Check sheet for the drawn part. Datum: minimum x, y, z corner. Units: mm. Coordinates: 2 decimals unless noted, no trailing zeros. Order: outer loops, then holes, each group sorted by start corner. A loop starts at its lowest first (then second) coordinate and runs counter-clockwise, first axis right, second up. Notation, with made-up numbers: (13.5, -12) -> (67.5, -12) arc R23 ccw to (67.5, 8) -> close; hole circle Ø6 at (52, 24). An arc over 180 degrees is marked (long way). Answer as CSV lines item,"result".
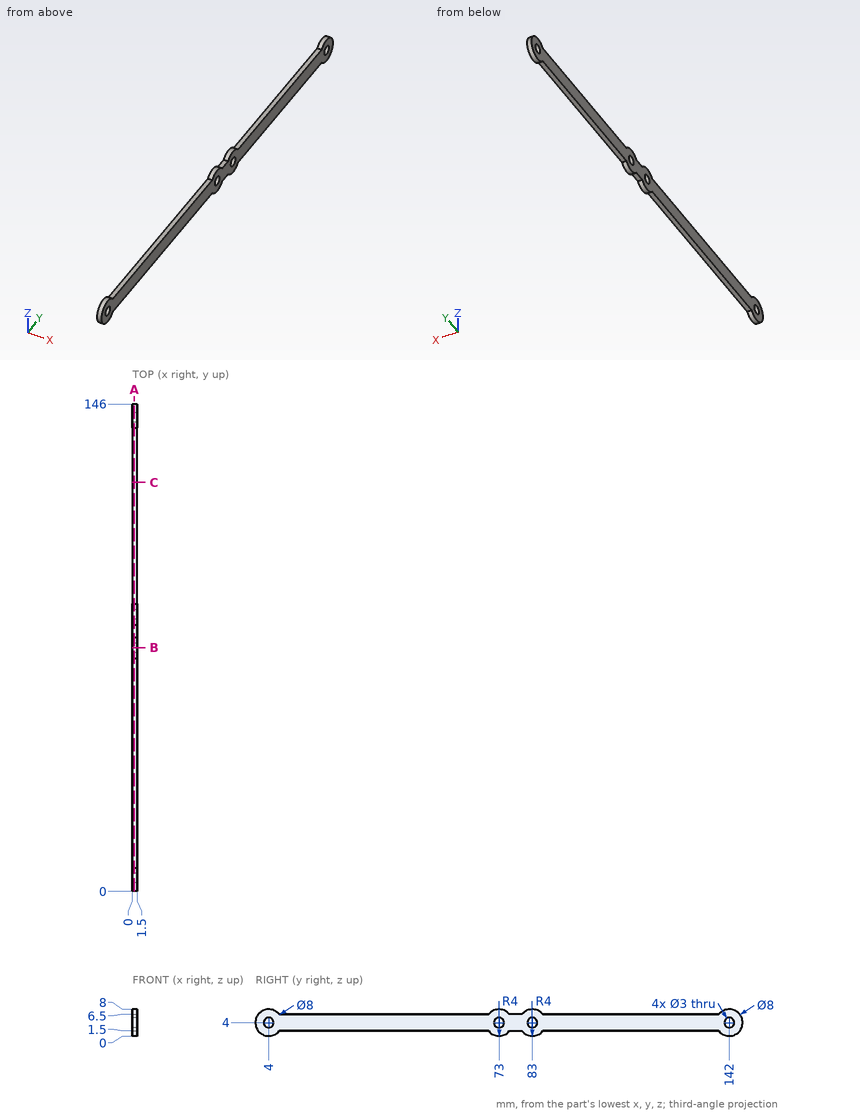
Item 1: Section check C-C, the plane y = 122.5. Record the boundary of the cut face in (x, z), plus the area to 3 significant figures.
Answer list:
outline,"(0, 1.5) -> (1.5, 1.5) -> (1.5, 6.5) -> (0, 6.5) -> close"
area,"7.50 mm2"
Item 2: Depth check by flat-ended pin: pin 1 Ø2.5 at (y, z) = (83, 4) entering from +X (3 decimals). Enter the tip coordinate at first touch or a pass-through.
Answer list:
pin 1,"through"
Item 3: Section check A-A, the plane x = 0.6. Record the boundary of the cut face in (y, z), plus the area to 3 significant figures.
Answer list:
outline,"(7.12, 1.5) -> (69.88, 1.5) arc R4 ccw to (76.12, 1.5) -> (79.88, 1.5) arc R4 ccw to (86.12, 1.5) -> (138.88, 1.5) arc R4 ccw (long way) to (138.88, 6.5) -> (86.12, 6.5) arc R4 ccw to (79.88, 6.5) -> (76.12, 6.5) arc R4 ccw to (69.88, 6.5) -> (7.12, 6.5) arc R4 ccw (long way) to start; hole circle Ø3 at (4, 4); hole circle Ø3 at (73, 4); hole circle Ø3 at (83, 4); hole circle Ø3 at (142, 4)"
area,"751 mm2"
Item 4: Section check B-B, the plane y = 73. Record the boundary of the cut face in (x, z).
Answer list:
outline,"(0, 0) -> (1.5, 0) -> (1.5, 2.5) -> (0, 2.5) -> close; (0, 5.5) -> (1.5, 5.5) -> (1.5, 8) -> (0, 8) -> close"
Item 5: Thickness scan on line 1 (Y direction, x = 1.2, z = 3.75); line 2 (Y direction, x = 1.45, z = 3.25); line 3 (Y direction, x = 1.15, z = 7.25). Record the ranges inside material, lowest first.
Answer list:
line 1,"0.01 to 2.52, 5.48 to 71.52, 74.48 to 81.52, 84.48 to 140.52, 143.48 to 145.99"
line 2,"0.07 to 2.7, 5.3 to 71.7, 74.3 to 81.7, 84.3 to 140.7, 143.3 to 145.93"
line 3,"1.67 to 6.33, 70.67 to 75.33, 80.67 to 85.33, 139.67 to 144.33"
